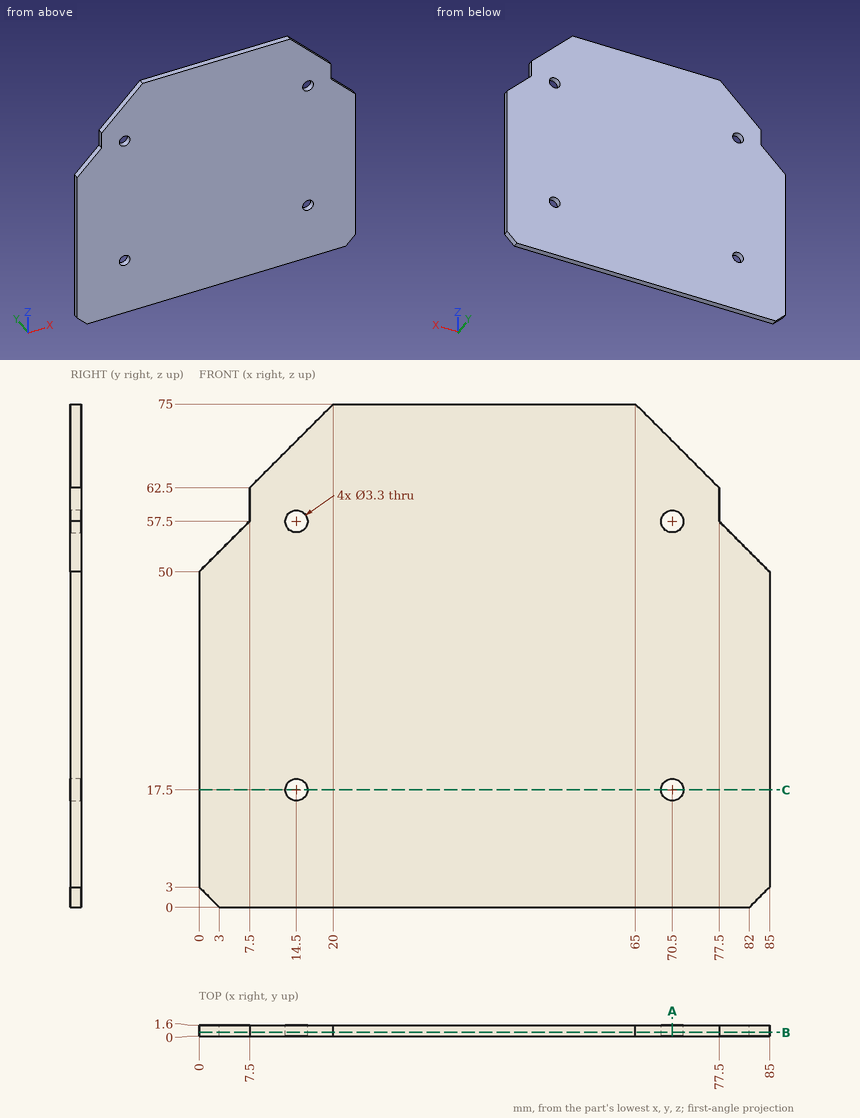
Input: dimensioned drawing with shaded views. Units: mm. Origin: part minimum x, y, z. Round coordinates to 2 decimals unless told otherwise and drop trailing zeros. Order: outer loops, then holes, each group sorted by start corner. A loop starts at its lowest first (then second) coordinate and runs counter-clockwise, first axis right, second up. Notation, with made-up numbers: M -20.5,80 L -5.5,80 A16 cw -5.5,91 Z; hole C -13.5,-10 d1. An arc over 180 degrees is marked long. Use one line per item in the form item = value. Start each with the question number.
Q1. Cut plane A-A (x = 70.5). Return loops of the section in (y, z), and give its area (3 significant figures).
Q2. Cut plane C-C (z = 17.5). Return loops of the section in (x, y), and give its area (3 significant figures).
Q3. Pin query (flat end, axial travel): pin 1 Ø3 at (x, z) = (14.5, 17.5) entering from +Y. Return the tip coordinate at first contact, or that it passes through.
Q4. Cut plane B-B (y = 0.55). Return loops of the section in (x, z).
Q5. Material intervals for line 1 (X direction, y = 0.55, z = 17.5); line 2 (X direction, y = 0.9, z = 57.5); line 3 (X direction, y = 0.5, z = 62.5), sorted ascending. Write a range as [from, to].
Geometry results:
q1.outline = M 0,0 L 1.6,0 L 1.6,15.85 L 0,15.85 Z; M 0,19.15 L 1.6,19.15 L 1.6,55.85 L 0,55.85 Z; M 0,59.15 L 1.6,59.15 L 1.6,69.5 L 0,69.5 Z
q1.area = 101 mm^2
q2.outline = M 0,0 L 12.85,0 L 12.85,1.6 L 0,1.6 Z; M 16.15,0 L 68.85,0 L 68.85,1.6 L 16.15,1.6 Z; M 72.15,0 L 85,0 L 85,1.6 L 72.15,1.6 Z
q2.area = 125 mm^2
q3.pin_1 = through
q4.outline = M 0,3 L 3,0 L 82,0 L 85,3 L 85,50 L 77.5,57.5 L 77.5,62.5 L 65,75 L 20,75 L 7.5,62.5 L 7.5,57.5 L 0,50 Z; hole C 14.5,17.5 d3.3; hole C 14.5,57.5 d3.3; hole C 70.5,17.5 d3.3; hole C 70.5,57.5 d3.3
q5.line_1 = [0, 12.85], [16.15, 68.85], [72.15, 85]
q5.line_2 = [7.5, 12.85], [16.15, 68.85], [72.15, 77.5]
q5.line_3 = [7.5, 77.5]
